```python
from build123d import *

# Parameters (mm, degrees)
SKETCH1_R           = 2.5
SKETCH1_R_2         = 2.55
SKETCH1_R_3         = 3.5685
BOSS_EXTRUDE1_DEPTH = 3.175


with BuildPart() as part:
    # Sketch1 → Boss-Extrude1 (new body)
    with BuildSketch(Plane(origin=(0, 0, 0), x_dir=(0, -1, 0), z_dir=(-1, 0, 0))):
        with BuildLine():
            Line((-80, 35), (-80, -35))
            ThreePointArc((-80, -35), (-77.071067812, -42.071067812), (-70, -45))
            Line((-70, -45), (70, -45))
            ThreePointArc((70, -45), (77.071067812, -42.071067812), (80, -35))
            Line((80, -35), (80, 35))
            ThreePointArc((80, 35), (77.071067812, 42.071067812), (70, 45))
            Line((70, 45), (-70, 45))
            ThreePointArc((-70, 45), (-77.071067812, 42.071067812), (-80, 35))
        make_face()
        with Locations(Location((50, 32.3, 0), (0, 0, 270))):
            Circle(SKETCH1_R, mode=Mode.SUBTRACT)
        with Locations(Location((50, -32.3, 0), (0, 0, 270))):
            Circle(SKETCH1_R, mode=Mode.SUBTRACT)
        with Locations(Location((-50, 32.3, 0), (0, 0, 270))):
            Circle(SKETCH1_R, mode=Mode.SUBTRACT)
        with Locations(Location((-50, -32.3, 0), (0, 0, 270))):
            Circle(SKETCH1_R, mode=Mode.SUBTRACT)
        with Locations(Location((10, 0, 0), (0, 0, 270))):
            Circle(SKETCH1_R_2, mode=Mode.SUBTRACT)
        with Locations(Location((-10, 0, 0), (0, 0, 270))):
            Circle(SKETCH1_R_2, mode=Mode.SUBTRACT)
        with Locations(Location((-20, 10, 0), (0, 0, 270))):
            Circle(SKETCH1_R_2, mode=Mode.SUBTRACT)
        with Locations(Location((-20, -10, 0), (0, 0, 270))):
            Circle(SKETCH1_R_2, mode=Mode.SUBTRACT)
        with Locations(Location((20, 10, 0), (0, 0, 270))):
            Circle(SKETCH1_R_2, mode=Mode.SUBTRACT)
        with Locations(Location((20, -10, 0), (0, 0, 270))):
            Circle(SKETCH1_R_2, mode=Mode.SUBTRACT)
        with Locations(Location((-70, 10, 0), (0, 0, 270))):
            Circle(SKETCH1_R, mode=Mode.SUBTRACT)
        with Locations(Location((70, 10, 0), (0, 0, 270))):
            Circle(SKETCH1_R, mode=Mode.SUBTRACT)
        with Locations(Location((-70, -10, 0), (0, 0, 270))):
            Circle(SKETCH1_R, mode=Mode.SUBTRACT)
        with Locations(Location((70, -10, 0), (0, 0, 270))):
            Circle(SKETCH1_R, mode=Mode.SUBTRACT)
        with Locations(Location((10, -32.3, 0), (0, 0, 270))):
            Circle(SKETCH1_R, mode=Mode.SUBTRACT)
        with Locations(Location((10, 32.3, 0), (0, 0, 270))):
            Circle(SKETCH1_R, mode=Mode.SUBTRACT)
        with Locations(Location((-10, 32.3, 0), (0, 0, 270))):
            Circle(SKETCH1_R, mode=Mode.SUBTRACT)
        with Locations(Location((-32.3, -32.3, 0), (0, 0, 270))):
            Circle(SKETCH1_R_3, mode=Mode.SUBTRACT)
        with Locations(Location((-32.3, 0, 0), (0, 0, 270))):
            Circle(SKETCH1_R_3, mode=Mode.SUBTRACT)
        with Locations(Location((-32.3, 32.3, 0), (0, 0, 270))):
            Circle(SKETCH1_R_3, mode=Mode.SUBTRACT)
        with Locations(Location((32.3, 32.3, 0), (0, 0, 270))):
            Circle(SKETCH1_R, mode=Mode.SUBTRACT)
        with Locations(Location((32.3, -32.3, 0), (0, 0, 270))):
            Circle(SKETCH1_R, mode=Mode.SUBTRACT)
        with Locations(Location((-10, -32.3, 0), (0, 0, 270))):
            Circle(SKETCH1_R, mode=Mode.SUBTRACT)
        with Locations(Location((0, 10, 0), (0, 0, 270))):
            Circle(SKETCH1_R, mode=Mode.SUBTRACT)
        with Locations(Location((0, -10, 0), (0, 0, 270))):
            Circle(SKETCH1_R, mode=Mode.SUBTRACT)
        with Locations(Location((70, 32.3, 0), (0, 0, 270))):
            Circle(SKETCH1_R_3, mode=Mode.SUBTRACT)
        with Locations(Location((0, 32.3, 0), (0, 0, 270))):
            Circle(SKETCH1_R_3, mode=Mode.SUBTRACT)
        with Locations(Location((-70, 32.3, 0), (0, 0, 270))):
            Circle(SKETCH1_R_3, mode=Mode.SUBTRACT)
        with Locations(Location((-70, -32.3, 0), (0, 0, 270))):
            Circle(SKETCH1_R, mode=Mode.SUBTRACT)
        with Locations(Location((70, -32.3, 0), (0, 0, 270))):
            Circle(SKETCH1_R, mode=Mode.SUBTRACT)
        with Locations(Location((0, -32.3, 0), (0, 0, 270))):
            Circle(SKETCH1_R, mode=Mode.SUBTRACT)
    extrude(amount=-BOSS_EXTRUDE1_DEPTH)


solid = part.part
```
Geometry: final body of the model. Coordinates: model frame, mm. Round coordinates to 2 decimals unless told otherwise and drop trailing zeros. Order: outer loops, then holes, each group sorted by start corner. A loop starts at its lowest first (then second) coordinate and runs counter-clockwise, first axis right, second up. Notation, with made-up numbers: M -29.5,-38.75 L -4.5,-38.75 A28 ccw -4.5,-7.75 Z; hole C 9,62.25 d10. An arc over 180 degrees is marked long. One line per item, written item: value.
(1) Cut plane A-A (y = -10). Return the cut outline in (x, z) (3 decimals), and give its area (3 significant figures).
Result sheet:
outline: M 0,-45 L 3.175,-45 L 3.175,-34.8 L 0,-34.8 Z; M 0,-29.8 L 3.175,-29.8 L 3.175,-2.55 L 0,-2.55 Z; M 0,2.55 L 3.175,2.55 L 3.175,29.8 L 0,29.8 Z; M 0,34.8 L 3.175,34.8 L 3.175,45 L 0,45 Z
area: 238 mm2
(2) Line query: probe 1 along Y at (x, z) = (1.3, -10); probe 2 along Z at (x, y) = (1.3, -70); probe 3 along Z at (x, y) = (0.9, -20). Output: solid intervals per line, ascending. Write a range as [from, to].
Result sheet:
probe 1: [-80, -72.5], [-67.5, -22.55], [-17.45, -2.5], [2.5, 17.45], [22.55, 67.5], [72.5, 80]
probe 2: [-45, -34.8], [-29.8, -12.5], [-7.5, 7.5], [12.5, 28.73], [35.87, 45]
probe 3: [-45, -12.55], [-7.45, 7.45], [12.55, 45]
(3) Cut plane B-B (y = -50). Return the cut outline in (x, z) (3 decimals).
Result sheet:
outline: M 0,-45 L 3.175,-45 L 3.175,-34.8 L 0,-34.8 Z; M 0,-29.8 L 3.175,-29.8 L 3.175,29.8 L 0,29.8 Z; M 0,34.8 L 3.175,34.8 L 3.175,45 L 0,45 Z
(4) Cut plane D-D (z = 40). Return the cut outline in (x, y) (3 decimals), and give its area (3 significant figures).
Result sheet:
outline: M 0,-78.66 L 3.175,-78.66 L 3.175,78.66 L 0,78.66 Z
area: 499 mm2
(5) Pin query (flat end, axial travel): P1, Ø4, axis at y = -50, z = -32.3, coming from the +X side. Return the tip coordinate at first contact, or that it passes through.
Result sheet:
P1: through
(6) Cut plane C-C (x = 1.65). Give the number of separate pieces and of enclosed holes in the cut face, and give its area (3 significant figures).
Result sheet:
separate pieces: 1
enclosed holes: 31
area: 13,600 mm2
